Input: part model. Units: mm. Frame: model coordinates. A direction names the side the tool comes from. Coordinates: 2 decimals unless noted, no trailing zeros. Order: outer loops, then holes, each group sorted by start corner. A loop starts at its lowest first (then second) coordinate and runs counter-clockwise, first axis right, second up. Notation, with made-up numbers: M 1,-12.75 L 41,-12.75 A12 ccw 41,6.25 Z; hole C 57.25,67.5 d8. An arc over 180 degrees is marked long. One line per item, written item: value.
```python
from build123d import *

# Parameters (mm, degrees)
BOSS_EXTRUDE1_DEPTH                 = 5
SKETCH3_W                           = 6
SKETCH3_H                           = 6
BOSS_EXTRUDE2_DEPTH                 = 15
F_8_CLEARANCE_HOLE2_D               = 4.4958
F_8_CLEARANCE_HOLE2_DEPTH           = 17
F_8_CLEARANCE_HOLE2_TIP             = 1.350674586
F_8_CLEARANCE_HOLE2_ON_FACE_2_D     = 4.4958
F_8_CLEARANCE_HOLE2_ON_FACE_2_DEPTH = 17
F_8_CLEARANCE_HOLE2_ON_FACE_2_TIP   = 1.350674586
SKETCH17_R                          = 0.625
CUT_EXTRUDE1_DEPTH                  = 30


with BuildPart() as part:
    # Sketch1 → Boss-Extrude1 (new body)
    with BuildSketch(Plane(origin=(0, 0, 0), x_dir=(1, 0, 0), z_dir=(0, 1, 0))):
        Polygon((-14.338976611, 0), (110.661023389, 0), (110.661023389, 55), (8.161023389, 55), (-14.338976611, 55), align=None)
    extrude(amount=BOSS_EXTRUDE1_DEPTH)

    # Sketch3 → Boss-Extrude2 (add)
    with BuildSketch(Plane(origin=(0, 0, 0), x_dir=(-1, 0, 0), z_dir=(0, -1, 0))):
        with Locations((-1.161023389, 44.75)):
            Rectangle(SKETCH3_W, SKETCH3_H)
        with Locations((-1.161023389, 10.25)):
            Rectangle(SKETCH3_W, SKETCH3_H)
        with Locations((-15.161023389, 44.934631069)):
            Rectangle(SKETCH3_W, SKETCH3_H)
        with Locations((-15.161023389, 10.240172473)):
            Rectangle(SKETCH3_W, SKETCH3_H)
    extrude(amount=BOSS_EXTRUDE2_DEPTH)

    # #8 Clearance Hole2
    with Locations(Plane(origin=(-1.838976611, -11, -44.75), x_dir=(0, 0, -1), z_dir=(-1, 0, 0))):
        with Locations((0, 0), (-34.5, 0)):
            Hole(F_8_CLEARANCE_HOLE2_D / 2, depth=F_8_CLEARANCE_HOLE2_DEPTH)
            with Locations((0, 0, -(F_8_CLEARANCE_HOLE2_DEPTH + F_8_CLEARANCE_HOLE2_TIP / 2))):  # 118° drill point
                Cone(0, F_8_CLEARANCE_HOLE2_D / 2, F_8_CLEARANCE_HOLE2_TIP, mode=Mode.SUBTRACT)

    # #8 Clearance Hole2 on face 2
    with Locations(Plane(origin=(18.161023389, -11, -44.934631069), x_dir=(0, 0, 1), z_dir=(1, 0, 0))):
        with Locations((0, 0), (34.694458596, 0)):
            Hole(F_8_CLEARANCE_HOLE2_ON_FACE_2_D / 2, depth=F_8_CLEARANCE_HOLE2_ON_FACE_2_DEPTH)
            with Locations((0, 0, -(F_8_CLEARANCE_HOLE2_ON_FACE_2_DEPTH + F_8_CLEARANCE_HOLE2_ON_FACE_2_TIP / 2))):  # 118° drill point
                Cone(0, F_8_CLEARANCE_HOLE2_ON_FACE_2_D / 2, F_8_CLEARANCE_HOLE2_ON_FACE_2_TIP, mode=Mode.SUBTRACT)

    # Sketch17 → Cut-Extrude1 (cut)
    with BuildSketch(Plane(origin=(110.661023389, 0, 0), x_dir=(0, 0, -1), z_dir=(1, 0, 0))):
        with Locations((27.5, 3.712457307)):
            Circle(SKETCH17_R)
    extrude(amount=-CUT_EXTRUDE1_DEPTH, mode=Mode.SUBTRACT)


solid = part.part
```
(1) First-contact query: pin 1 (3 mm diameter, centred on y = -8.5, z = -44, fed in from +X); pin 2 (5 mm diameter, centred on x = 1.5, y = -9.5, fed in from +Z); pin 3 (3 mm diameter, centred on y = -4, z = -45, fed in from -X). Flat tips, straight axial feed; report the tip coordinate or a pass-through.
Data:
pin 1: stops at x = 18.16
pin 2: stops at z = -7.25
pin 3: stops at x = -1.84
(2) Cut plane D-D on z = -38. Output: boundary loops of the cut face in (x, y).
Data:
outline: M -14.34,0 L 110.66,0 L 110.66,5 L -14.34,5 Z
(3) Ray query, line 1 (Z direction, x = -0.5, y = -11); line 2 (Z direction, x = 0.5, y = -5.75); line 3 (Y direction, x = 1.75, z = -44.75). Return the intervals inside material, ascending. Write a range as from..to.
Data:
line 1: z = -47.75..-47, -42.5..-41.75, -13.25..-12.5, -8..-7.25
line 2: z = -47.75..-41.75, -13.25..-7.25
line 3: y = -15..-13.25, -8.75..5
(4) Cut plane C-C on x = 89.5. Output: boundary loops of the cut face in (y, z) (3 decimals).
Data:
outline: M 0,-55 L 5,-55 L 5,0 L 0,0 Z; hole C 3.712,-27.5 d1.25
(5) Cut plane A-A on y = -5.25. Output: boundary loops of the cut face in (x, z), plus the area to 3 significant figures.
Data:
outline: M -1.84,-47.75 L 4.16,-47.75 L 4.16,-41.75 L -1.84,-41.75 Z; M -1.84,-13.25 L 4.16,-13.25 L 4.16,-7.25 L -1.84,-7.25 Z; M 12.16,-47.93 L 18.16,-47.93 L 18.16,-41.93 L 12.16,-41.93 Z; M 12.16,-13.24 L 18.16,-13.24 L 18.16,-7.24 L 12.16,-7.24 Z
area: 144 mm2
(6) Access query for faces 1 (the flat face through (12.161, -7, -45)), 2 (the flat face through (1, -7, -7.25)), 3 (the cylindrical face through (2.64, -11.049, -7.993)), 4 (the cylindrical face through (2.64, -10.95, -47.18)). Directions: +Z, -Z, +X, -X, +Y, -Y. A direction counts if a zero-diameter tool reaches every point of the face in a straight line with its end or side. Return the directions, or none.
Data:
face 1: +Z, -Z, -Y
face 2: +Z, +X, -X, -Y
face 3: +X, -X
face 4: +X
(7) Cut plane B-B on y = -11. Give the number of separate pieces and of enclosed holes in the cut face, plus the area to 3 significant figures.
Data:
separate pieces: 8
enclosed holes: 0
area: 34.9 mm2
(8) Draft query along X for faces 5 (the flat face through (15, -7, -13.24)), 6 (the flat face through (-1.839, -7, -45)), 7 (the flat face through (4.161, -7, -10)). Return one class per face: released by +X, released by -X, zero draft, split by the parting line, or undercut.
Data:
face 5: zero draft
face 6: released by -X
face 7: undercut
